from build123d import *

# Parameters (mm, degrees)
SKETCH1_W           = 95
SKETCH1_H           = 50
BOSS_EXTRUDE1_DEPTH = 8
SKETCH2_W           = 55
SKETCH2_H           = 15
CUT_EXTRUDE1_DEPTH  = 55.270157545
SKETCH3_R           = 3.25
CUT_EXTRUDE2_DEPTH  = 55.270157545
SKETCH4_R           = 10.25
CUT_EXTRUDE3_DEPTH  = 6
FILLET1_R           = 5
SKETCH5_R           = 2
CUT_EXTRUDE4_DEPTH  = 55.270157545
CUT_EXTRUDE5_DEPTH  = 3
FILLET2_R           = 5


with BuildPart() as part:
    # Sketch1 → Boss-Extrude1 (new body)
    with BuildSketch(Plane(origin=(0, 0, 0), x_dir=(1, 0, 0), z_dir=(0, 1, 0))):
        Rectangle(SKETCH1_W, SKETCH1_H)
    extrude(amount=BOSS_EXTRUDE1_DEPTH)

    # Sketch2 → Cut-Extrude1 (cut, through all)
    with BuildSketch(Plane(origin=(0, 8, 0), x_dir=(1, 0, 0), z_dir=(0, 1, 0))):
        with Locations((0, 17.5)):
            Rectangle(SKETCH2_W, SKETCH2_H)
    extrude(amount=-CUT_EXTRUDE1_DEPTH, mode=Mode.SUBTRACT)

    # Sketch3 → Cut-Extrude2 (cut, through all)
    with BuildSketch(Plane(origin=(0, 8, 0), x_dir=(1, 0, 0), z_dir=(0, 1, 0))):
        with Locations(Location((0, 2, 0), (0, 0, 270))):
            Circle(SKETCH3_R)
    extrude(amount=-CUT_EXTRUDE2_DEPTH, mode=Mode.SUBTRACT)

    # Sketch4 → Cut-Extrude3 (cut)
    with BuildSketch(Plane.XZ):
        with Locations((0, -2)):
            Circle(SKETCH4_R)
    extrude(amount=-CUT_EXTRUDE3_DEPTH, mode=Mode.SUBTRACT)

    # Fillet1
    fillet1_edges = [part.edges().sort_by_distance(p)[0] for p in [
        (6.408002809, 3, -10),
        (-6.408002809, 3, -10),
    ]]
    fillet(fillet1_edges, radius=FILLET1_R)

    # Sketch5 → Cut-Extrude4 (cut, through all)
    with BuildSketch(Plane(origin=(0, 8, 0), x_dir=(1, 0, 0), z_dir=(0, 1, 0))):
        with Locations(Location((42.5, 20, 0), (0, 0, 270))):
            Circle(SKETCH5_R)
        with Locations(Location((42.5, -22, 0), (0, 0, 270))):
            Circle(SKETCH5_R)
        with Locations(Location((-42.5, -22, 0), (0, 0, 90))):
            Circle(SKETCH5_R)
        with Locations(Location((-42.5, 20, 0), (0, 0, 90))):
            Circle(SKETCH5_R)
    extrude(amount=-CUT_EXTRUDE4_DEPTH, mode=Mode.SUBTRACT)

    # Sketch6 → Cut-Extrude5 (cut)
    with BuildSketch(Plane(origin=(0, 8, 0), x_dir=(1, 0, 0), z_dir=(0, 1, 0))):
        with BuildLine():
            Line((-42.5, -18), (-47.5, -18))
            Line((-47.5, -18), (-47.5, -25))
            Line((-47.5, -25), (-45.145751311, -25))
            ThreePointArc((-45.145751311, -25), (-38.758342613, -23.414213562), (-42.5, -18))
        make_face()
        with BuildLine():
            Line((47.5, -25), (45.145751311, -25))
            ThreePointArc((45.145751311, -25), (38.758342613, -23.414213562), (42.5, -18))
            Line((42.5, -18), (47.5, -18))
            Line((47.5, -18), (47.5, -25))
        make_face()
        with BuildLine():
            Line((-42.5, 16), (-47.5, 16))
            Line((-47.5, 16), (-47.5, 25))
            Line((-47.5, 25), (-38.5, 25))
            Line((-38.5, 25), (-38.5, 20))
            ThreePointArc((-38.5, 20), (-39.671572875, 17.171572875), (-42.5, 16))
        make_face()
        with BuildLine():
            Line((42.5, 16), (47.5, 16))
            Line((47.5, 16), (47.5, 25))
            Line((47.5, 25), (38.5, 25))
            Line((38.5, 25), (38.5, 20))
            ThreePointArc((38.5, 20), (39.671572875, 17.171572875), (42.5, 16))
        make_face()
    extrude(amount=-CUT_EXTRUDE5_DEPTH, mode=Mode.SUBTRACT)

    # Fillet2
    fillet2_edges = [part.edges().sort_by_distance(p)[0] for p in [
        (-47.5, 6.5, 18),
        (-39.854248689, 6.5, 25),
        (47.5, 6.5, 18),
        (39.854248689, 6.5, 25),
        (-47.5, 2.5, 25),
        (47.5, 2.5, 25),
        (47.5, 2.5, -25),
        (47.5, 6.5, -16),
        (38.5, 6.5, -25),
        (-47.5, 2.5, -25),
        (-38.5, 6.5, -25),
        (-47.5, 6.5, -16),
    ]]
    fillet(fillet2_edges, radius=FILLET2_R - 0.0001)  # a hair under: the kernel refuses the full size


solid = part.part
Design review of the part built by this model. Coordinates are the model's own, in mm. A direction names the side the tool comes from. Give positions to 0.01 mm unless a question says otherwise; leave off trailing zeros. Write each loop counter-clockwise with the first axis right and the second up, starting at its lowest first coordinate (ties: lowest second). Pieces come first, ordered by that corner, then holes. Notation, with made-up numbers: M -37.75,-38.75 L -18.75,-38.75 A17 ccw -18.75,-19.75 Z; hole C -13.75,49 d6. An arc over 180 degrees is marked long. Answer as a JSON object with one key per item and string values. Group by question number.
1) For line 1 along Z through (x, y) = (-42.5, 2.9); line 2 along X through (y, z) = (3, -20); line 3 along X through (y, z) = (2.3, -2), list the stretches that pass through material, from the lowest coordinate up.
2) Clearance check with flat-ended pins moving along their axes: pin 1 Ø2.5 at (x, y) = (-1.5, 4.5) entering from -Z; pin 2 Ø3.5 at (x, z) = (42.5, 22) entering from -Y; pin 3 Ø5.5 at (x, z) = (5, 2.5) entering from -Y; pin 4 Ø4 at (x, z) = (-43, -19) entering from +Y. State where each tip first meets the part, or that it passes through.
3) We need section D-D (x = 37). Give the boundary of the cut face in (y, z).
4) We need section A-A (x = 0). Give the boundary of the cut face in (y, z), and give its area (4 significant figures).
5) We need section B-B (z = -2). Give the boundary of the cut face in (x, y), and give its area (3 significant figures).
6) We need section C-C (y = 2.75). Give the boundary of the cut face in (x, z).
7) Mouldability with a two-part tool opening along X and no side actions: class faces 1 (the face through (-27.5, 4, -17)), 2 (the face through (47.5, 3, 0)), 3 (the face through (-1, 0, 11)), 4 (the face through (11.045, 2.958, -8.121)) as released by +X, released by -X, zero draft, split by the parting line, or undercut.
8) Tool access review of faces 5 (the face through (46, 6.48, 16.57)), 6 (the face through (46.07, 6.48, -14.5)), 7 (the face through (-36.88, 6.52, 23.88)): name each direction out of +Z, -Z, +X, -X, +Y, -Y from which nothing blocks a thin tool from reaching the whole face with its end or side.
Answer key:
{
 "1": {"line 1": "z = -25 to -22, -18 to 20, 24 to 25", "line 2": "x = -47.5 to -44.5, -40.5 to -27.5, 27.5 to 40.5, 44.5 to 47.5", "line 3": "x = -47.5 to -10.25, 10.25 to 47.5"},
 "2": {"pin 1": "stops at z = 7.87", "pin 2": "passes through", "pin 3": "stops at y = 6", "pin 4": "stops at y = 5"},
 "3": {"outline": "M 0,-25 L 5,-25 L 5,-23.57 L 8,-23.57 L 8,23.78 L 5,23.78 L 5,25 L 0,25 Z"},
 "4": {"outline": "M 0,8.25 L 6,8.25 L 6,1.25 L 8,1.25 L 8,25 L 0,25 Z; M 6,-10 L 8,-10 L 8,-5.25 L 6,-5.25 Z", "area": "157.5 mm²"},
 "5": {"outline": "M -47.5,0 L -10.25,0 L -10.25,6 L -3.25,6 L -3.25,8 L -47.5,8 Z; M 3.25,6 L 10.25,6 L 10.25,0 L 47.5,0 L 47.5,8 L 3.25,8 Z", "area": "624 mm²"},
 "6": {"outline": "M -47.5,-20 A5 ccw -42.5,-25 L -27.5,-25 L -27.5,-10 L -14.95,-10 A5 ccw -10.05,-4.02 A10.25 cw long 10.05,-4.02 A5 ccw 14.95,-10 L 27.5,-10 L 27.5,-25 L 42.5,-25 A5 ccw 47.5,-20 L 47.5,20 A5 ccw 42.5,25 L -42.5,25 A5 ccw -47.5,20 Z; hole C -42.5,-20 d4; hole C -42.5,22 d4; hole C 42.5,-20 d4; hole C 42.5,22 d4"},
 "7": {"face 1": "undercut", "face 2": "released by +X", "face 3": "zero draft", "face 4": "undercut"},
 "8": {"face 5": "+Z, +X, +Y", "face 6": "-Z, +X, +Y", "face 7": "+Z, -X, +Y"}
}
